from build123d import *

# Parameters (mm, degrees)
SKETCH2_W                = 20
SKETCH2_H                = 6.020278893
BOSS_EXTRUDE1_DEPTH      = 4
FILLET1_R                = 1
M3_CLEARANCE_HOLE1_D     = 3.4
M3_CLEARANCE_HOLE1_DEPTH = 16.5
M3_CLEARANCE_HOLE1_TIP   = 1.021463052


with BuildPart() as part:
    # Sketch2 → Boss-Extrude1 (new body)
    with BuildSketch(Plane.XY.offset(133.365661293)):
        with Locations((-21.327645728, 38.168378797)):
            Rectangle(SKETCH2_W, SKETCH2_H)
    extrude(amount=BOSS_EXTRUDE1_DEPTH)

    # Fillet1
    fillet1_edges = [part.edges().sort_by_distance(p)[0] for p in [
        (-31.327645728, 41.178518244, 135.365661293),
        (-11.327645728, 41.178518244, 135.365661293),
        (-11.327645728, 35.158239351, 135.365661293),
        (-31.327645728, 35.158239351, 135.365661293),
    ]]
    fillet(fillet1_edges, radius=FILLET1_R)

    # M3 Clearance Hole1
    with Locations(Plane.XY.offset(137.365661293)):
        with Locations((-28.827645728, 37.778518244), (-13.827645728, 37.778518244)):
            Hole(M3_CLEARANCE_HOLE1_D / 2, depth=M3_CLEARANCE_HOLE1_DEPTH)
            with Locations((0, 0, -(M3_CLEARANCE_HOLE1_DEPTH + M3_CLEARANCE_HOLE1_TIP / 2))):  # 118° drill point
                Cone(0, M3_CLEARANCE_HOLE1_D / 2, M3_CLEARANCE_HOLE1_TIP, mode=Mode.SUBTRACT)


solid = part.part
Geometry check sheet. Reference: the model listing, model coordinates, mm. Give positions to 0.01 mm unless a question says otherwise; leave off trailing zeros. Loops run counter-clockwise (first coordinate to the right, second up) from the corner with the lowest first, then second, coordinate; pieces in that order, holes last.
(1) Section check B-B on z = 135.15. Record the cut outline in (x, y), then the cut area to 3 significant figures.
From the geometry:
outline: (-31.33, 36.16) arc R1 ccw to (-30.33, 35.16) - (-12.33, 35.16) arc R1 ccw to (-11.33, 36.16) - (-11.33, 40.18) arc R1 ccw to (-12.33, 41.18) - (-30.33, 41.18) arc R1 ccw to (-31.33, 40.18) - close; hole circle Ø3.4 at (-28.83, 37.78); hole circle Ø3.4 at (-13.83, 37.78)
area: 101 mm2
(2) Section check A-A on x = -30. Record the cut outline in (y, z), then the cut area to 3 significant figures.
From the geometry:
outline: (35.16, 133.37) - (36.55, 133.37) - (36.55, 137.37) - (35.16, 137.37) - close; (39.01, 133.37) - (41.18, 133.37) - (41.18, 137.37) - (39.01, 137.37) - close
area: 14.2 mm2
(3) Section check C-C on y = 38. Record the cut outline in (x, z), then the cut area to 3 significant figures.
From the geometry:
outline: (-31.33, 133.37) - (-30.51, 133.37) - (-30.51, 137.37) - (-31.33, 137.37) - close; (-27.14, 133.37) - (-15.51, 133.37) - (-15.51, 137.37) - (-27.14, 137.37) - close; (-12.14, 133.37) - (-11.33, 133.37) - (-11.33, 137.37) - (-12.14, 137.37) - close
area: 53.0 mm2
(4) Section check D-D on x = -27.75. Record the cut outline in (y, z), then the cut area to 3 significant figures.
From the geometry:
outline: (35.16, 133.37) - (36.46, 133.37) - (36.46, 137.37) - (35.16, 137.37) - close; (39.09, 133.37) - (41.18, 133.37) - (41.18, 137.37) - (39.09, 137.37) - close
area: 13.6 mm2
(5) Thickness scan on L1, parallel to X at y = 36.5, z = 136.9; L2, parallel to X at y = 39.25, z = 134.5; L3, parallel to Y at x = -30.25, z = 136.05. Record the ranges inside material, lowest first.
From the geometry:
L1: x = -31.33 to -29.95, -27.71 to -14.95, -12.71 to -11.33
L2: x = -31.33 to -29.68, -27.98 to -14.68, -12.98 to -11.33
L3: y = 35.16 to 36.85, 38.71 to 41.18
(6) Release check for a two-part mould opening along X. For faces 1 (the cylindrical face through (-11.613, 40.878, 135.394)), 2 (the cylindrical face through (-31.042, 35.459, 135.394)), 3 (the cylindrical face through (-27.13, 37.85, 135.34)) record: released by +X, released by -X, zero draft, split by the parting line, or undercut.
From the geometry:
face 1: released by +X
face 2: released by -X
face 3: undercut
